Geometry check sheet. Reference: the model listing, model coordinates, mm. A direction names the side the tool comes from. Round coordinates to 2 decimals unless told otherwise and drop trailing zeros. Loops run counter-clockwise (first coordinate to the right, second up) from the corner with the lowest first, then second, coordinate; pieces in that order, holes last. Notation, with made-up numbers: (7, 34) -> (62, 34) arc R20 ccw to (62, 63) -> close; hole circle Ø10 at (36, -7). An arc over 180 degrees is marked (long way). Use a Markdown table: item, result. Add a question column.
Q1. Gauge pin test, flat ends, axial feed: P1, Ø4.5, axis at x = 1, z = 21, coming from the -Y side; P2, Ø4.5, axis at x = -1, z = 19, coming from the -Y side; P3, Ø2.5, axis at x = 0.5, z = 20.5, coming from the +Y side; P4, Ø2, axis at y = 36, z = 17.5, coming from the +X side. Record the tip position at first contact, or that the pin passes through.
Q2. Set-up check for faces 4 (the face through (0, 0, 13)), 5 (the face through (-7.012, 0, 22)), 6 (the face through (-1, 1, 31)): record each of +Z, -Z, +X, -X, +Y, -Y from which the full face is reachable in a straight line by a thin tool's end or side.
Q3. Sectioned sample at D-D, the plane z = 9.5. Enter the section's corners in (x, y) (3 decimals).
Q4. Release check for a two-part mould opening along Y. For faces 1 (the face through (0, -27.057, 22)), 2 (the face through (-27.676, 21.221, 9.49)), 3 (the face through (22, 37, 27)) record: released by +Y, released by -Y, zero draft, split by the parting line, or undercut.
Q5. Sectioned sample at B-B, the plane x = 0. Enter the section's corners in (y, z) (3 decimals), then the cut area to 3 significant figures.
Q6. Sectioned sample at A-A, the plane z = 16. Give the number of separate pieces and of enclosed holes in the cut face, then the cut area to 3 significant figures.
Q7. Material ranges on L1, parallel to Y at x = 0, z = 7 (3 decimals); L2, parallel to X at y = -6, z = 22.5; L3, parallel to Y at x = 0, z = 22, recorded low to high.
Autodesk Inventor part; units mm, degrees
ref_plane "YZ Plane" through (0, 0, 0) normal (1, 0, 0) x (0, 1, 0)
ref_plane "XZ Plane" through (0, 0, 0) normal (0, 1, 0) x (-1, 0, 0)
ref_plane "XY Plane" through (0, 0, 0) normal (0, 0, 1) x (1, 0, 0)
sketch "Boceto1" plane through (0, 0, 0) normal (0, 0, 1) x (1, 0, 0)
  circle A0 centre (0, 0) radius 30.5
  circle A1 centre (0, 0) radius 34.875
  dimension "d0" = 61
  dimension "d1" = 69.75
extrude "Extrusión1" add sketch "Boceto1" along normal blind 27
sketch "Boceto2" plane through (0, 0, 27) normal (0, 0, 1) x (1, 0, 0)
  circle A0 centre (0, 0) radius 35.0049
  circle A1 centre (0, 0) radius 30.5
  circle A2 centre (0, 0) radius 49.5
  dimension "d4" = 19
extrude "Extrusión2" add sketch "Boceto2" along normal blind 4 contours A0 | A2
sketch "Boceto3" plane through (0, 0, 27) normal (0, 0, -1) x (-1, 0, 0)
  point P0 (0, 0)
fillet "Empalme1" radius 7.75 1 edges at (-34.875, 0, 27)
sketch "Boceto4" plane through (0, 0, 0) normal (0, 0, -1) x (-1, 0, 0)
  circle A0 centre (0, 0) radius 31.639
  line L0 (-6.5155, -30.9609) -> (6.5155, -30.9609)
  line L1 (6.5155, -30.9609) -> (6.5155, 30.9609)
  line L2 (6.5155, 30.9609) -> (-6.5155, 30.9609)
  line L3 (-6.5155, 30.9609) -> (-6.5155, -30.9609)
  line L4 (-6.5155, -30.9609) -> (6.5155, 30.9609) construction
  line L5 (6.5155, -30.9609) -> (-6.5155, 30.9609) construction
sketch "Boceto5" plane through (0, 0, 31) normal (0, 0, 1) x (1, 0, 0)
  line L0 (-7.0125, -31.5254) -> (7.0125, -31.5254)
  line L1 (7.0125, -31.5254) -> (7.0125, 31.5254)
  line L2 (7.0125, 31.5254) -> (-7.0125, 31.5254)
  line L3 (-7.0125, 31.5254) -> (-7.0125, -31.5254)
  line L4 (-7.0125, -31.5254) -> (7.0125, 31.5254) construction
  line L5 (7.0125, -31.5254) -> (-7.0125, 31.5254) construction
  line L6 (-4.4061, -27.0572) -> (4.4061, -27.0572)
  line L7 (4.4061, -27.0572) -> (4.4061, 27.0572)
  line L8 (4.4061, 27.0572) -> (-4.4061, 27.0572)
  line L9 (-4.4061, 27.0572) -> (-4.4061, -27.0572)
  line L10 (-4.4061, -27.0572) -> (4.4061, 27.0572) construction
  line L11 (4.4061, -27.0572) -> (-4.4061, 27.0572) construction
  line L12 (-4.4061, -10.4257) -> (4.4061, -10.4257)
  line L13 (4.4061, -10.4257) -> (4.4061, 10.4257)
  line L14 (4.4061, 10.4257) -> (-4.4061, 10.4257)
  line L15 (-4.4061, 10.4257) -> (-4.4061, -10.4257)
  line L16 (-4.4061, -10.4257) -> (4.4061, 10.4257) construction
  line L17 (4.4061, -10.4257) -> (-4.4061, 10.4257) construction
  point P0 (0, 0)
extrude "Extrusión3" add sketch "Boceto5" against normal blind 18 contours L3 L2 L1 L0 | L9 L14 L7 L12
properties part number "Base_robot_base_3DPrint"
Values:
| question | item | result |
|---|---|---|
| 1 | P1 | y = -35.97 |
| 1 | P2 | y = -35.13 |
| 1 | P3 | y = 35.29 |
| 1 | P4 | through |
| 2 | face 4 | -Z |
| 2 | face 5 | +Z, -Z |
| 2 | face 6 | +Z, +X, -X, +Y, -Y |
| 3 | outline | circle Ø69.75 at (0, 0); hole circle Ø61 at (0, 0) |
| 4 | face 1 | undercut |
| 4 | face 2 | split by the parting line |
| 4 | face 3 | zero draft |
| 5 | outline | (-49.5, 27) -> (-42.625, 27) arc R7.75 cw to (-34.875, 19.25) -> (-34.875, 0) -> (-30.5, 0) -> (-30.5, 13) -> (-27.057, 13) -> (-27.057, 31) -> (-49.5, 31) -> close; (-10.426, 13) -> (10.426, 13) -> (10.426, 31) -> (-10.426, 31) -> close; (27.057, 13) -> (30.5, 13) -> (30.5, 0) -> (34.875, 0) -> (34.875, 19.25) arc R7.75 cw to (42.625, 27) -> (49.5, 27) -> (49.5, 31) -> (27.057, 31) -> close |
| 5 | area | 913 mm^2 |
| 6 | separate pieces | 1 |
| 6 | enclosed holes | 4 |
| 6 | area | 1,450 mm^2 |
| 7 | L1 | -34.875 to -30.5, 30.5 to 34.875 |
| 7 | L2 | -35.08 to -29.9, -7.01 to 7.01, 29.9 to 35.08 |
| 7 | L3 | -35.38 to -27.06, -10.43 to 10.43, 27.06 to 35.38 |
